from build123d import *

# Parameters (mm, degrees)
SKETCH_2_W = 151
SKETCH_2_H = 126
SKETCH_1_W = 134
SKETCH_1_H = 110
SKETCH_3_W = 143.875710796
SKETCH_3_H = 118.62726712
SKETCH_4_W = 125.407231672
SKETCH_4_H = 101.536444544


with BuildPart() as part:
    # 草图2 → 放样2 section 0
    with BuildSketch(Plane.XY.offset(67)):
        with Locations((67, 55)):
            Rectangle(SKETCH_2_W, SKETCH_2_H)
    # 草图1 → 放样2 section 1
    with BuildSketch(Plane.XY):
        with Locations((67, 55)):
            Rectangle(SKETCH_1_W, SKETCH_1_H)
    loft()

    # 草图3 → 切除-放样3 section 0
    with BuildSketch(Plane.XY.offset(67)):
        with Locations((67, 55)):
            Rectangle(SKETCH_3_W, SKETCH_3_H)
    # 草图4 → 切除-放样3 section 1
    with BuildSketch(Plane(origin=(0, 0, 1), x_dir=(-1, 0, 0), z_dir=(0, 0, -1))):
        with Locations((-67, 55)):
            Rectangle(SKETCH_4_W, SKETCH_4_H)
    loft(mode=Mode.SUBTRACT)


solid = part.part
Can you work these out from the model? Positions are in its coordinate system, mm. Round coordinates to 2 decimals unless told otherwise and drop trailing zeros. Write item = value, one per line. Start each with the question number.
(1) If we mould it in two halves opening along X, with no side actions, what happens to faces 1 (the face through (72, 116, 67)), 2 (the face through (65, 55, 1))? For each: released by +X, released by -X, zero draft, split by the parting line, or undercut.
(2) If I drill on probe 1 along Z at (x, y) = (34, 62); probe 2 along X at (y, z) = (8, 11); probe 3 along X at (y, z) = (61.5, 17), over which ranges is the centre line in solid material (lowest first)? Write a range as [from, to].
(3) For P1, Ø10, axis at y = 92.5, z = 12, coming from the +X side; P2, Ø2, axis at y = 101, z = 9.5, coming from the -X side; P3, Ø4, axis at y = 81.5, z = 51, coming from the +X side, each with a flat end and sliding along its axis, tell me the tip position at first contact or that it passes through.
Ans:
q1.face_1 = zero draft
q1.face_2 = undercut
q2.probe_1 = [0, 1]
q2.probe_2 = [-1.4, 2.9], [131.1, 135.4]
q2.probe_3 = [-2.16, 2.06], [131.94, 136.16]
q3.P1 = 136.16
q3.P2 = -1.33
q3.P3 = 140.72
